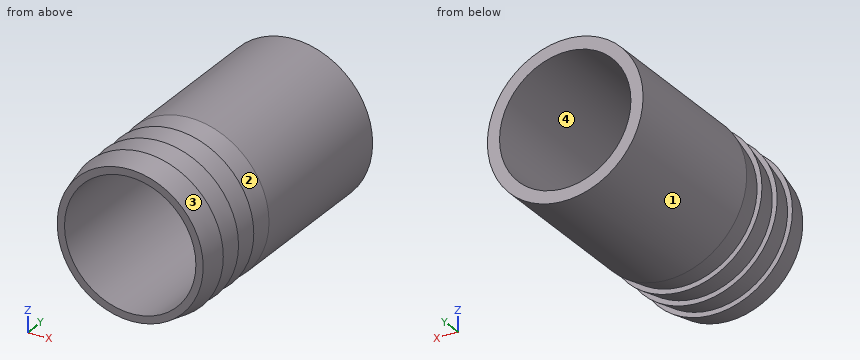
from build123d import *

# Parameters (mm, degrees)
SKETCH1_R           = 16
SKETCH1_R_2         = 13.5
BOSS_EXTRUDE1_DEPTH = 54


with BuildPart() as part:
    # Sketch1 → Boss-Extrude1 (new body)
    with BuildSketch(Plane(origin=(0, 0, 0), x_dir=(1, 0, 0), z_dir=(0, 1, 0))):
        Circle(SKETCH1_R)
        Circle(SKETCH1_R_2, mode=Mode.SUBTRACT)
    extrude(amount=BOSS_EXTRUDE1_DEPTH)

    # Sketch2 → Cut-Revolve2 (revolve, cut)
    with BuildSketch(Plane.XY):
        Polygon((16, 15), (16, 20), (15, 15), align=None)
        Polygon((16, 0), (16, 5), (15, 0), align=None)
        Polygon((16, 5), (16, 10), (15, 5), align=None)
        Polygon((16, 10), (16, 15), (15, 10), align=None)
    revolve(axis=Axis((0, 0, 0), (0, 1, 0)), mode=Mode.SUBTRACT)


solid = part.part
Can you work these out from the model? Positions are in its coordinate system, mm. Face numbers are marked on the shaded views. A direction names the side the tool comes from. Give positions to 0.01 mm unless a question says otherwise; leave off trailing zeros. Loops run counter-clockwise (first coordinate to the right, second up) from the corner with the lowest first, then second, coordinate; pieces in that order, holes last. Notation, with made-up numbers: (61.25, 65.5) -> (89.25, 65.5) arc R14 ccw to (89.25, 92.5) -> close; hole circle Ø7 at (45.25, 6.5). An arc over 180 degrees is marked (long way). Return JSON: item names as keys, results as strings.
Q1. I want a section at B-B, the plane z = 0. List the corners of the cut face in (x, y) for me.
Checks:
{"outline": "(-16, 5) -> (-15, 0) -> (-13.5, 0) -> (-13.5, 54) -> (-16, 54) -> (-16, 20) -> (-15, 15) -> (-16, 15) -> (-15, 10) -> (-16, 10) -> (-15, 5) -> close; (13.5, 0) -> (15, 0) -> (16, 5) -> (15, 5) -> (16, 10) -> (15, 10) -> (16, 15) -> (15, 15) -> (16, 20) -> (16, 54) -> (13.5, 54) -> close"}
Q2. For pin 1 Ø1.5 at (x, y) = (10.5, 22.5) entering from +Z; pin 2 Ø6 at (x, y) = (7, 36.5) entering from -Z; pin 3 Ø10 at (y, z) = (18.5, -9.5) entering from +X, each with a flat end and sliding along its axis, tell me the tip position at first contact or that it passes through.
Checks:
{"pin 1": "stops at z = 12.69", "pin 2": "stops at z = -15.49", "pin 3": "stops at x = 15.28"}
Q3. I need wall thicknesses on probe 1 along Z at (x, y) = (0, 25); probe 2 along X at (y, z) = (44.5, -2.5). Which ranges of each line are inside material? Lowest first, please.
Checks:
{"probe 1": "z = -16 to -13.5, 13.5 to 16", "probe 2": "x = -15.8 to -13.27, 13.27 to 15.8"}
Q4. I want a section at D-D, the plane y = 49.5. List the corners of the cut face in (x, z) for me.
Checks:
{"outline": "circle Ø32 at (0, 0); hole circle Ø27 at (0, 0)"}
Q5. On a 3-axis mill with a long thin cutter (end or side, diameter ignored), from which of +Z, -Z, +X, -X, +Y, -Y can I reach the whole of each face in a straight line? I mean the marked faces 1 and 2. Say none if no direction works.
Checks:
{"face 1": "+Y, -Y", "face 2": "none"}
Q6. We'd pull the mould along X, two halves only. Please class the marked faces 3 and 4: released by +X, released by -X, zero draft, split by the parting line, or undercut.
Checks:
{"face 3": "split by the parting line", "face 4": "undercut"}
Q7. I want a section at A-A, the plane x = 0. List the corners of the cut face in (y, z) for me.
Checks:
{"outline": "(0, -15) -> (5, -16) -> (5, -15) -> (10, -16) -> (10, -15) -> (15, -16) -> (15, -15) -> (20, -16) -> (54, -16) -> (54, -13.5) -> (0, -13.5) -> close; (0, 13.5) -> (54, 13.5) -> (54, 16) -> (20, 16) -> (15, 15) -> (15, 16) -> (10, 15) -> (10, 16) -> (5, 15) -> (5, 16) -> (0, 15) -> close"}
Q8. I want a section at C-C, the plane y = 13. List the corners of the cut face in (x, z) for me, then the cut area to 3 significant figures.
Checks:
{"outline": "circle Ø31.2 at (0, 0); hole circle Ø27 at (0, 0)", "area": "192 mm2"}
